Could you check a few things on this model? Use its own coordinates, in mm. A direction names the side the tool comes from. Round coordinates to 2 decimals unless told otherwise and drop trailing zeros. Write each loop counter-clockwise with the first axis right and the second up, starting at its lowest first coordinate (ties: lowest second). Pieces come first, ordered by that corner, then holes.
Autodesk Inventor part; units mm, degrees
ref_plane "YZ Plane" through (0, 0, 0) normal (1, 0, 0) x (0, 1, 0)
ref_plane "XZ Plane" through (0, 0, 0) normal (0, 1, 0) x (-1, 0, 0)
ref_plane "XY Plane" through (0, 0, 0) normal (0, 0, 1) x (1, 0, 0)
sketch "Эскиз1" plane through (0, 0, 0) normal (0, 0, 1) x (1, 0, 0)
  circle A0 centre (0, 0) radius 2.5
  circle A1 centre (7.6, 7.6) radius 1.5
  circle A2 centre (-7.6, 7.6) radius 1.5
  circle A3 centre (-7.6, -7.6) radius 1.5
  circle A4 centre (7.6, -7.6) radius 1.5
  arc A5 (-8.5, 10) -> (-10, 8.5) centre (-8.5, 8.5) ccw
  line L0 (-8.5, 10) -> (8.5, 10)
  line L1 (-10, -8.5) -> (-10, 8.5)
  line L2 (-10, -8.5) -> (-10, -3.95)
  arc A6 (-10, -8.5) -> (-8.5, -10) centre (-8.5, -8.5) ccw
  line L3 (-3.95, -10) -> (-8.5, -10)
  line L4 (8.5, -10) -> (-8.5, -10)
  arc A7 (8.5, -10) -> (10, -8.5) centre (8.5, -8.5) ccw
  line L5 (10, -3.95) -> (10, -8.5)
  line L6 (10, 8.5) -> (10, -8.5)
  arc A8 (10, 8.5) -> (8.5, 10) centre (8.5, 8.5) ccw
  line L7 (3.95, 10) -> (8.5, 10)
extrude "Выдавливание1" add sketch "Эскиз1" along normal blind 1 contours A0 | A1 | A2 | A3 | A4 | L0 A8 L6 L5 A7 L4 L3 A6 L1 A5
fillet "Сопряжение1" radius 0.5 8 edges at (-9.5607, -9.5607, 1) (0, -10, 1) (9.5607, -9.5607, 1) (10, -6.225, 1) (9.5607, 9.5607, 1) (6.225, 10, 1) (-9.5607, 9.5607, 1) (-10, -6.225, 1)
sketch "Эскиз2" plane through (0, 0, 0) normal (0, 0, -1) x (-1, 0, 0)
  circle A0 centre (0, 0) radius 2.5
extrude "Выдавливание2" add sketch "Эскиз2" along normal blind 3
fillet "Сопряжение2" radius 1 1 edges at (2.5, 0, -3)
sketch "Эскиз3" plane through (0, 0, 0) normal (0, 0, -1) x (-1, 0, 0)
  line L0 (-10, -8.5) -> (-10, 8.5)
  line L1 (0, 0) -> (0, -8.5)
  arc A0 (6.2205, -3.7242) -> (6.8074, -3.9673) centre (6.8074, -3.1373) ccw
  line L2 (8.0499, -3.9673) -> (6.8074, -3.9673)
  line L3 (8.0267, -3.2811) -> (8.0407, -3.2952)
  line L4 (4.6459, 0.629) -> (4.6459, 2.1594)
  arc A1 (5.1321, 3.3332) -> (4.6459, 2.1594) centre (6.3059, 2.1594) ccw
  line L5 (6.8074, 4.6647) -> (8.0267, 4.6647)
  line L6 (6.2205, -3.7242) -> (5.1321, -2.6359)
  arc A2 (4.6459, -1.4621) -> (5.1321, -2.6359) centre (6.3059, -1.4621) ccw
  arc A3 (6.8074, 4.6647) -> (6.2205, 4.4216) centre (6.8074, 3.8347) ccw
  line L7 (5.1321, 3.3332) -> (6.2205, 4.4216)
  arc A4 (4.6459, 0.0684) -> (4.6431, 0.1025) centre (4.4384, 0.0684) ccw
  line L8 (4.6459, -1.4621) -> (4.6459, 0.629)
  arc A5 (4.6431, 0.5948) -> (4.6459, 0.629) centre (4.4384, 0.629) ccw
  line L9 (8.0499, -3.9673) -> (8.0267, -2.2602)
  line L10 (7.9913, 0.3493) -> (4.6459, 0.3493)
  line L11 (9.9996, 5.5485) -> (10, 5.5489)
  line L12 (8.0267, 2.9588) -> (8.0267, 4.6647)
  line L13 (8.0267, 2.9588) -> (10, 2.9588)
  line L14 (10, 8.5) -> (10, -8.5)
  line L15 (8.0267, -2.2602) -> (10, -2.2602)
  arc A6 (-6.8074, -3.9673) -> (-6.2205, -3.7242) centre (-6.8074, -3.1373) ccw
  line L16 (-8.0499, -3.9673) -> (-6.8074, -3.9673)
  line L17 (-8.0267, -3.2811) -> (-8.0407, -3.2952)
  line L18 (-6.2205, -3.7242) -> (-5.1321, -2.6359)
  arc A7 (-5.1321, -2.6359) -> (-4.6459, -1.4621) centre (-6.3059, -1.4621) ccw
  line L19 (-8.0499, -3.9673) -> (-8.0267, -2.2602)
  arc A8 (-4.6431, 0.1025) -> (-4.6459, 0.0684) centre (-4.4384, 0.0684) ccw
  line L20 (-4.6459, 0.629) -> (-4.6459, 2.1594)
  arc A9 (-4.6459, 2.1594) -> (-5.1321, 3.3332) centre (-6.3059, 2.1594) ccw
  line L21 (-6.8074, 4.6647) -> (-8.0267, 4.6647)
  line L22 (-7.9913, 0.3493) -> (-4.6459, 0.3493)
  arc A10 (-4.6459, 0.629) -> (-4.6431, 0.5948) centre (-4.4384, 0.629) ccw
  line L23 (-4.6459, -1.4621) -> (-4.6459, 0.629)
  line L24 (-9.9996, 5.5485) -> (-10, 5.5489)
  line L25 (-8.0267, 2.9588) -> (-8.0267, 4.6647)
  line L26 (-5.1321, 3.3332) -> (-6.2205, 4.4216)
  arc A11 (-6.2205, 4.4216) -> (-6.8074, 4.6647) centre (-6.8074, 3.8347) ccw
  line L27 (-8.0267, 2.9588) -> (-10, 2.9588)
  line L28 (-8.0267, -2.2602) -> (-10, -2.2602)
  point P0 (10, -4.8504)
  point P1 (-10, -4.8504)
extrude "Выдавливание3" add sketch "Эскиз3" along normal blind 3
properties part number "затычка"
Q1. On a 3-axis mill with a long thin cutter (end or side, diameter ignored), from which of +Z, -Z, +X, -X, +Y, -Y can I reach the whole of each face in a straight line? I mean faces 4 (the flat face through (-4.646, 0, -1)), 5 (the flat face through (-7, 4.665, -1)), 6 (the flat face through (5.684, -3.188, -1.479)). Say none if no direction works.
Q2. If I drill on L1, parallel to X at y = 1.75, z = -2.25; L2, parallel to X at y = -1.75, z = -0.25; L3, parallel to Z at x = -2.5, y = -1, over which ranges is the centre line in solid material (lowest first)?
Q3. I'm going to push flat-ended pins straight in: pin 1 Ø1 at (x, z) = (7.5, -1) entering from +Y; pin 2 Ø0.5 at (y, z) = (4, -1) entering from +X; pin 3 Ø1.6 at (x, z) = (8.5, -1.5) entering from -Y. Where does each tip first touch, or does it pass through?
Q4. We'd pull the mould along X, two halves only. Please class faces 1 (the flat face through (-5.7, 3.9, -1.5)), 2 (the flat face through (-9, -2.26, -1)), 3 (the flat face through (-8.027, 4, -1)): pulls with the +X half, pulls with the -X half, needs draft (parallel to the pull), parting line crosses it, or undercut.
Q5. Imagine slicing it at A-A, the plane z = -1.7. Count the separate pieces of the cut face and the enclosed holes in it, then the cut area to 3 significant figures.
Q6. Imagine slicing it at D-D, the plane x = 3.5. Write out the boundary of the cut face in (y, z), then the cut area to 3 significant figures.
Q7. Imagine slicing it at B-B, the plane x = 0. Write out the boundary of the cut face in (y, z), then the cut area to 3 significant figures.
Q8. Imagine slicing it at C-C, the plane y = 0. Write out the boundary of the cut face in (x, z).
Results found:
1. face 4: -Z, +Y, -Y
1. face 5: -Z, +X, -X, +Y
1. face 6: -Z, -Y
2. L1: x = -10 to -4.65, -1.74 to 1.74, 4.65 to 10
2. L2: x = -10 to -4.67, -1.79 to 1.79, 4.67 to 10
2. L3: z = 0 to 1
3. pin 1: stops at y = 4.66
3. pin 2: stops at x = 8.03
3. pin 3: stops at y = -3.97
4. face 1: undercut
4. face 2: needs draft
4. face 3: pulls with the -X half
5. separate pieces: 3
5. enclosed holes: 0
5. area: 91.7 mm2
6. outline: (-10, 0) - (10, 0) - (10, 0.5) arc R0.5 ccw to (9.5, 1) - (-9.5, 1) arc R0.5 ccw to (-10, 0.5) - close
6. area: 19.9 mm2
7. outline: (-10, 0) - (-2.5, 0) - (-2.5, -2) arc R1 ccw to (-1.5, -3) - (1.5, -3) arc R1 ccw to (2.5, -2) - (2.5, 0) - (10, 0) - (10, 0.5) arc R0.5 ccw to (9.5, 1) - (-9.5, 1) arc R0.5 ccw to (-10, 0.5) - close
7. area: 34.5 mm2
8. outline: (-10, -3) - (-4.65, -3) - (-4.65, 0) - (-2.5, 0) - (-2.5, -2) arc R1 ccw to (-1.5, -3) - (1.5, -3) arc R1 ccw to (2.5, -2) - (2.5, 0) - (4.65, 0) - (4.65, -3) - (10, -3) - (10, 0.5) arc R0.5 ccw to (9.5, 1) - (-9.5, 1) arc R0.5 ccw to (-10, 0.5) - close
